Geometry check sheet. Reference: drawing and pictorial views, mm from the part's lowest x, y, z. A direction names the side the tool comes from. Round coordinates to 2 decimals unless told otherwise and drop trailing zeros. Write each loop counter-clockwise with the first axis right and the second up, starting at its lowest first coordinate (ties: lowest second). Pieces come first, ordered by that corner, then holes. Notation, with made-up numbers: M 13,52.5 L 38,52.5 A23 ccw 38,89.5 Z; hole C 7.5,17.25 d3. An arc over 180 degrees is marked long. Answer in a Markdown table with one row per item.
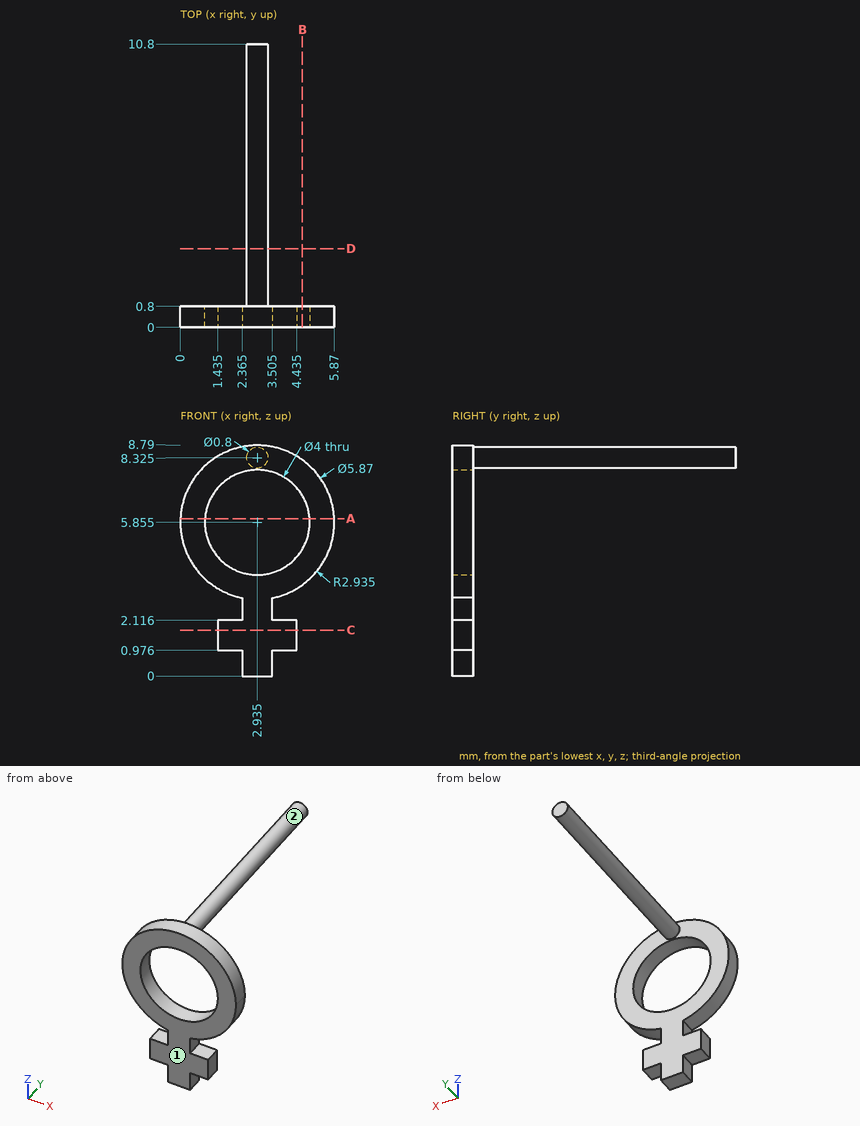
1. Section check D-D, the plane y = 3. Record the cut outline in (x, z) (1 decimal).
Found:
| item | result |
|---|---|
| outline | C 2.9,8.3 d0.8 |
2. Section check C-C, the plane z = 1.75. Record the cut outline in (x, y) (1 decimal).
Found:
| item | result |
|---|---|
| outline | M 1.4,0 L 4.4,0 L 4.4,0.8 L 1.4,0.8 Z |
3. Go/stop test with flat-tipped pins: pin 1 (1.8 mm diameter, centred on x = 2, z = 4, fed in from +Y); pin 2 (3 mm diameter, centred on x = 2.935, z = 5.855, fed in from +Y); pin 3 (2 mm diameter, centred on x = 3.5, y = 3, fed in from +Z) (1 decimal); pin 4 (0.9 mm diameter, centred on x = 4, y = 0.5, fed in from -Z). Record where each tip stops, or that it passes through.
Found:
| item | result |
|---|---|
| pin 1 | stops at y = 0.8 |
| pin 2 | passes through |
| pin 3 | stops at z = 8.7 |
| pin 4 | stops at z = 0.98 |
4. Access from +Z, -Z, +X, -X, +Y, -Y to the whole of each face (thin tool, end or side, straight path). Record for the marked faces 1 and 2.
Found:
| item | result |
|---|---|
| face 1 | +Z, -Z, +X, -X, -Y |
| face 2 | +Y |
5. Section check A-A, the plane z = 6. Record the cut outline in (x, y).
Found:
| item | result |
|---|---|
| outline | M 0,0 L 0.94,0 L 0.94,0.8 L 0,0.8 Z; M 4.93,0 L 5.87,0 L 5.87,0.8 L 4.93,0.8 Z |
6. Scan lines: L1, parallel to Y at x = 0.8, z = 5.75; L2, parallel to X at y = 0.75, z = 5.25. Record each from-to range of solid material in increasing order.
Found:
| item | result |
|---|---|
| L1 | y = 0 to 0.8 |
| L2 | x = 0.06 to 1.03, 4.84 to 5.81 |
7. Section check B-B, the plane x = 4.65. Record the cut outline in (y, z).
Found:
| item | result |
|---|---|
| outline | M 0,3.47 L 0.8,3.47 L 0.8,4.83 L 0,4.83 Z; M 0,6.88 L 0.8,6.88 L 0.8,8.24 L 0,8.24 Z |
